Source: CAD feature listing. Evaluate the final solid. Frame: model axes, mm. Give positions to 0.01 mm unless a question says otherwise; leave off trailing zeros. Order: outer loops, then holes, each group sorted by start corner. A loop starts at its lowest first (then second) coordinate and runs counter-clockwise, first axis right, second up.
from build123d import *

# Parameters (mm, degrees)
CAMERA_REMOVABLE_PANEL_W = 120
CAMERA_REMOVABLE_PANEL_H = 100
CAMERA_REMOVABLE_PANEL_R = 1.7
F_3MM_DEPTH              = 3


with BuildPart() as part:
    # 外形与孔位_camera_removable_panel → 板厚_3mm (new body)
    with BuildSketch(Plane.XY):
        with Locations((60, 50)):
            Rectangle(CAMERA_REMOVABLE_PANEL_W, CAMERA_REMOVABLE_PANEL_H)
        with Locations((10, 10)):
            Circle(CAMERA_REMOVABLE_PANEL_R, mode=Mode.SUBTRACT)
        with Locations((10, 90)):
            Circle(CAMERA_REMOVABLE_PANEL_R, mode=Mode.SUBTRACT)
        with Locations((110, 10)):
            Circle(CAMERA_REMOVABLE_PANEL_R, mode=Mode.SUBTRACT)
        with Locations((110, 90)):
            Circle(CAMERA_REMOVABLE_PANEL_R, mode=Mode.SUBTRACT)
    extrude(amount=F_3MM_DEPTH)


solid = part.part
(1) Section A-A, the plane x = 10. Return loops of the section in (y, z).
(2) Pin query (flat end, axial travel): pin 1 Ø12 at (x, y) = (87.5, 52) entering from -Z. Return the tip coordinate at first contact, or that it passes through.
(3) Draft query along Y for faces 1 (the flat face through (59, 100, 1)), 2 (the cylindrical face through (9.63, 8.34, 1.48)), 3 (the flat face through (59, 0, 1)), 4 (the flat face through (59, 51, 3)). Return one class per face: +Y half, -Y half, draft (parallel to the pull), parting line (faces both ways), or undercut.
(4) Section B-B, the plane y = 90. Return loops of the section in (x, z), plus the area to 3 significant figures.
(5) Line query: line 1 along Y through (x, z) = (110, 1.85); line 2 along X through (y, z) = (90, 2.35). Output: solid intervals per line, ascending.
Checks:
1. outline: (0, 0) - (8.3, 0) - (8.3, 3) - (0, 3) - close; (11.7, 0) - (88.3, 0) - (88.3, 3) - (11.7, 3) - close; (91.7, 0) - (100, 0) - (100, 3) - (91.7, 3) - close
2. pin 1: stops at z = 0
3. face 1: +Y half
3. face 2: undercut
3. face 3: -Y half
3. face 4: draft
4. outline: (0, 0) - (8.3, 0) - (8.3, 3) - (0, 3) - close; (11.7, 0) - (108.3, 0) - (108.3, 3) - (11.7, 3) - close; (111.7, 0) - (120, 0) - (120, 3) - (111.7, 3) - close
4. area: 340 mm2
5. line 1: y = 0 to 8.3, 11.7 to 88.3, 91.7 to 100
5. line 2: x = 0 to 8.3, 11.7 to 108.3, 111.7 to 120
